```python
from build123d import *

# Parameters (mm, degrees)
BOSS_EXTRUDE1_DEPTH          = 3
BOSS_EXTRU_1_DEPTH           = 30.6
ESQUISSE2_R                  = 1.0000000000000018
ENL_V_MAT_EXTRU_1_DEPTH      = 3
ESQUISSE3_R                  = 2.349999999999996
BOSS_EXTRU_2_DEPTH           = 3
ESQUISSE4_R                  = 2.5
ENL_V_MAT_EXTRU_2_DEPTH      = 42.11398788733586
ENL_V_MAT_EXTRU_3_DEPTH      = 5
ENL_V_MAT_EXTRU_3_DEPTH_BACK = 1.5
ESQUISSE6_R                  = 0.4999999999999987
ESQUISSE6_R_2                = 0.5000000000000008
ESQUISSE6_R_3                = 0.49999999999999967
ESQUISSE6_R_4                = 3.749999999999999
ENL_V_MAT_EXTRU_4_DEPTH      = 3


with BuildPart() as part:
    # Sketch1 → Boss-Extrude1 (new body)
    with BuildSketch(Plane(origin=(0, 0, 0), x_dir=(1, 0, 0), z_dir=(0, 1, 0))):
        with BuildLine():
            Line((19, 15), (16.00000000000001, 15))
            ThreePointArc((16.00000000000001, 15.000000000000007), (8.070475080311514, 14.151517110035783), (0.5000000000000107, 11.644487847162011))
            ThreePointArc((0.5000000000000098, 11.64448784716201), (-6.999999999999976, -4.4e-16), (0.5000000000000098, -11.644487847162011))
            ThreePointArc((0.5000000000000107, -11.644487847162011), (8.070475080311514, -14.151517110035783), (16.00000000000001, -15.000000000000007))
            Line((16.00000000000001, -15), (19, -15))
            Line((19, -15), (19, 15))
        make_face()
    extrude(amount=-BOSS_EXTRUDE1_DEPTH)

    # Esquisse1 → Boss.-Extru.1 (add)
    with BuildSketch(Plane(origin=(0, 0, 0), x_dir=(1, 0, 0), z_dir=(0, 1, 0))):
        Polygon((19, 15), (16.000000000000007, 15), (16.00000000000001, -15), (19.000000000000004, -15), align=None)
    extrude(amount=BOSS_EXTRU_1_DEPTH)

    # Esquisse2 → Enlèv. mat.-Extru.1 (cut)
    with BuildSketch(Plane(origin=(0, 30.6, 0), x_dir=(1, 0, 0), z_dir=(0, 1, 0))):
        with Locations(Location((17.500000000000004, 10, 0), (0, 0, 270))):
            Circle(ESQUISSE2_R)
        with Locations(Location((17.500000000000004, -10, 0), (0, 0, 270))):
            Circle(ESQUISSE2_R)
    extrude(amount=-ENL_V_MAT_EXTRU_1_DEPTH, mode=Mode.SUBTRACT)

    # Esquisse3 → Boss.-Extru.2 (add)
    with BuildSketch(Plane(origin=(0, 0, 0), x_dir=(1, 0, 0), z_dir=(0, 1, 0))):
        with Locations(Location((0, 0, 0), (0, 0, 270))):
            Circle(ESQUISSE3_R)
    extrude(amount=BOSS_EXTRU_2_DEPTH)

    # Esquisse4 → Enlèv. mat.-Extru.2 (cut, through all)
    with BuildSketch(Plane.ZY.offset(-16.000000000000007)):
        with Locations((0, 15.3)):
            Circle(ESQUISSE4_R)
    extrude(amount=-ENL_V_MAT_EXTRU_2_DEPTH, mode=Mode.SUBTRACT)

    # Esquisse5 → Enlèv. mat.-Extru.3 (cut, two sides: drawn at the far end of the back side and taken through both)
    with BuildSketch(Plane.ZY.offset(-16.000000000000007).offset(-ENL_V_MAT_EXTRU_3_DEPTH_BACK)):
        with BuildLine():
            Line((-2.8000000000001206, 12.805506063347845), (-1.9323091258538179, 1.1685931981230362))
            add(Edge.make_bspline(
                [(-1.9323091258538179, 1.1685931981230362), (-1.9048352156569601, 0.8027138716048543), (-1.7460527055675423, 0.47250804579621575), (-1.5874431867330887, 0.14266197447294557), (-1.3185847338688517, -0.10715488116746878), (-1.0505560477953044, -0.3562007373159315), (-0.7091686681940543, -0.4905620157021409), (-0.3678310237411564, -0.6249037196151552), (-1.5634e-13, -0.6249999999988765), (0.3661752794111309, -0.6250958469887595), (0.7080076723836786, -0.4910181757340655), (1.0487343876149366, -0.35737418689144385), (1.3178512419643233, -0.1078357174129213), (1.5861375320152837, 0.14093261173257243), (1.745511479884174, 0.4713841828126921), (1.9047478532446405, 0.8015505020492266), (1.932309125853515, 1.1685931981230258)],
                knots=[0, 0, 0, 0.125, 0.125, 0.25, 0.25, 0.375, 0.375, 0.5, 0.5, 0.625, 0.625, 0.75, 0.75, 0.875, 0.875, 1, 1, 1], degree=2))
            Line((1.932309125853515, 1.1685931981230258), (2.7999999999998786, 12.80550606334783))
            ThreePointArc((2.7999999999998786, 12.80550606334783), (3.7499999999998854, 15.300000000001111), (2.799999999999892, 17.794493936654398))
            Line((2.799999999999892, 17.794493936654398), (1.9323091258535894, 29.43140680187921))
            add(Edge.make_bspline(
                [(1.9323091258535894, 29.43140680187921), (1.9048352156568606, 29.797286128395676), (1.746052705567315, 30.12749195420603), (1.587443186734994, 30.45733802552631), (1.318584733868623, 30.70715488116971), (1.0505560477969664, 30.956200737317417), (0.7091686681938255, 31.090562015704386), (0.36783102373777693, 31.224903719618656), (-7.308e-14, 31.225000000001117), (-0.36617527942078804, 31.22509584698975), (-0.7080076723839066, 31.091018175736306), (-1.0487343876225454, 30.957374186888348), (-1.3178512419645536, 30.70783571741516), (-1.586137532016866, 30.45906738826691), (-1.745511479884403, 30.128615817189548), (-1.9047478532448734, 29.798449497952962), (-1.932309125853744, 29.431406801879216)],
                knots=[0, 0, 0, 0.125, 0.125, 0.25, 0.25, 0.375, 0.375, 0.5, 0.5, 0.625, 0.625, 0.75, 0.75, 0.875, 0.875, 1, 1, 1], degree=2))
            Line((-1.932309125853744, 29.431406801879216), (-2.8000000000001077, 17.794493936654412))
            ThreePointArc((-2.8000000000001077, 17.794493936654412), (-3.7500000000001132, 15.300000000001132), (-2.8000000000001206, 12.805506063347845))
        make_face()
    extrude(amount=ENL_V_MAT_EXTRU_3_DEPTH + ENL_V_MAT_EXTRU_3_DEPTH_BACK, mode=Mode.SUBTRACT)

    # Esquisse6 → Enlèv. mat.-Extru.4 (cut)
    with BuildSketch(Plane(origin=(19, 0, 0), x_dir=(0, 0, -1), z_dir=(1, 0, 0))):
        with Locations((7.86e-14, 30.20000000000113)):
            Circle(ESQUISSE6_R)
        with Locations((8.389e-14, 28.200000000001125)):
            Circle(ESQUISSE6_R)
        with Locations((8.917e-14, 26.200000000001125)):
            Circle(ESQUISSE6_R)
        with Locations((9.445e-14, 24.200000000001122)):
            Circle(ESQUISSE6_R_2)
        with Locations((9.974e-14, 22.200000000001125)):
            Circle(ESQUISSE6_R_3)
        with Locations((1.0502e-13, 20.200000000001125)):
            Circle(ESQUISSE6_R)
        with Locations((1.309e-13, 10.400000000001125)):
            Circle(ESQUISSE6_R_3)
        with Locations((1.3619e-13, 8.400000000001125)):
            Circle(ESQUISSE6_R_3)
        with Locations((1.4147e-13, 6.400000000001126)):
            Circle(ESQUISSE6_R_3)
        with Locations((1.4675e-13, 4.400000000001127)):
            Circle(ESQUISSE6_R_3)
        with Locations((1.5204e-13, 2.4000000000011252)):
            Circle(ESQUISSE6_R_3)
        with Locations((1.5732e-13, 0.4000000000011234)):
            Circle(ESQUISSE6_R_3)
        with Locations((1.1848e-13, 15.300000000001125)):
            Circle(ESQUISSE6_R_4)
    extrude(amount=-ENL_V_MAT_EXTRU_4_DEPTH, mode=Mode.SUBTRACT)


solid = part.part
```
Geometry check sheet. Reference: the model listing, model coordinates, mm. A direction names the side the tool comes from. Round coordinates to 2 decimals unless told otherwise and drop trailing zeros. Loops run counter-clockwise (first coordinate to the right, second up) from the corner with the lowest first, then second, coordinate; pieces in that order, holes last. Notation, with made-up numbers: (18.5, 51) -> (58.5, 51) arc R21 cw to (58.5, 80) -> close; hole circle Ø5 at (60.25, 70). An arc over 180 degrees is marked (long way). Use a Markdown table: item, result.
(1) Go/stop test with flat-tipped pins: P1, Ø5, axis at x = -0.5, z = 1, coming from the +Y side; P2, Ø11.5, axis at x = 9.5, z = 2.5, coming from the +Y side; P3, Ø2, axis at y = 25.5, z = -12, coming from the -X side; P4, Ø4.5, axis at y = 15.3, z = 0, coming from the -X side. Record where each tip stops, or that it passes through.
Calculated:
| item | result |
|---|---|
| P1 | y = 3 |
| P2 | y = 0 |
| P3 | x = 16 |
| P4 | through |
(2) Mould release check, pull along X, two halves, no side actions. Record for faces 6 (the flat face through (17, 30.6, 8)), 7 (the flat face through (17.5, 6, 1)), 8 (the flat face through (19, 14, 4)): released by +X, released by -X, zero draft, split by the parting line, or undercut.
Calculated:
| item | result |
|---|---|
| face 6 | zero draft |
| face 7 | undercut |
| face 8 | released by +X |
(3) Scan lines: probe 1 along Y at (x, z) = (10.75, 10); probe 2 along X at (y, z) = (25.5, 5); probe 3 along X at (y, z) = (8, -1). Record each from-to range of solid material in increasing order.
Calculated:
| item | result |
|---|---|
| probe 1 | -3 to 0 |
| probe 2 | 16 to 19 |
| probe 3 | 17.5 to 19 |
(4) Sectioned sample at C-C (x = 0). Enter the section's corners in (y, z), then the cut area to 3 significant figures.
Calculated:
| item | result |
|---|---|
| outline | (-3, -11.4) -> (0, -11.4) -> (0, -2.35) -> (3, -2.35) -> (3, 2.35) -> (0, 2.35) -> (0, 11.4) -> (-3, 11.4) -> close |
| area | 82.5 mm² |
(5) Sectioned sample at A-A (y = 28.2). Enter the section's corners in (x, z).
Calculated:
| item | result |
|---|---|
| outline | (16, -15) -> (19, -15) -> (19, -0.5) -> (17.5, -0.5) -> (17.5, -2.02) -> (16, -2.02) -> close; (16, 2.02) -> (17.5, 2.02) -> (17.5, 0.5) -> (19, 0.5) -> (19, 15) -> (16, 15) -> close; hole circle Ø2 at (17.5, -10); hole circle Ø2 at (17.5, 10) |
(6) Sectioned sample at D-D (z = -12.5). Enter the section's corners in (x, y).
Calculated:
| item | result |
|---|---|
| outline | (2.54, -3) -> (19, -3) -> (19, 30.6) -> (16, 30.6) -> (16, 0) -> (2.54, 0) -> close |
(7) Sectioned sample at B-B (y = 4.4). Enter the section's corners in (x, z), then the cut area to 3 significant figures.
Calculated:
| item | result |
|---|---|
| outline | (16, -15) -> (19, -15) -> (19, -0.5) -> (17.5, -0.5) -> (17.5, -2.17) -> (16, -2.17) -> close; (16, 2.17) -> (17.5, 2.17) -> (17.5, 0.5) -> (19, 0.5) -> (19, 15) -> (16, 15) -> close |
| area | 82.0 mm² |
(8) Set-up check for faces 1 (the cylindrical face through (18.261, 1.912, 0.108)), 2 (the cylindrical face through (18.261, 23.712, 0.108)), 3 (the flat face through (18, 27.6, -10)), 4 (the flat face through (16.76, 23.69, -2.36)), 5 (the flat face through (18, 14, -15)): record each of +Z, -Z, +X, -X, +Y, -Y from which the full face is reachable in a straight line by a thin tool's end or side.
Calculated:
| item | result |
|---|---|
| face 1 | +X |
| face 2 | +X, -X |
| face 3 | +Y |
| face 4 | -X |
| face 5 | -Z, +X, -X, +Y, -Y |
